For this review, take the finished solid that the model builds, in its own axes (mm). Face numbers are marked on the shaded views. A direction names the side the tool comes from. Round coordinates to 2 decimals unless told otherwise and drop trailing zeros. Order: outer loops, then holes, each group sorted by start corner. A loop starts at its lowest first (then second) coordinate and runs counter-clockwise, first axis right, second up. Notation, with made-up numbers: (54.25, 26.5) - (100.25, 26.5) arc R17 ccw to (100.25, 58.5) - close; hole circle Ø8 at (12, 7). An arc over 180 degrees is marked (long way). Write each question's results on one line, items separated by ' | '. Start each with the question number.
(1) Take a section at D-D, the plane y = -18. Give the boundary of the cut face in (x, z).
(2) Insertion check: pin 1 Ø1 at (y, z) = (2.5, 9) entering from +X; pin 2 Ø1 at (x, z) = (-17.5, 9) entering from -Y; pin 3 Ø1.5 at (x, y) = (5, -10) entering from -Z; pin 4 Ø3 at (x, z) = (-1.5, 5) entering from +Y. Each pin has a flat end and moves straight along its axis. Give the tip position at first contact, or say it passes through.
(3) Take a section at A-A, the plane x = 0. Give the boundary of the cut face in (y, z), plus the area to 3 significant figures.
(4) Take a section at C-C, the plane z = 10.75. Give the boundary of the cut face in (x, y), plus the area to 3 significant figures.
(5) For the marked faces 1, 2 and 3, list the 3-axis set-ups (+Z, -Z, +X, -X, +Y, -Y) from which the entire face can be reached by the end or side of a thin tool; tool diameter is ignored.
(6) Draft analysis for pull direction X (two halves, no side actions). For the marked faces 4, 5 and 6, state which applies: pulls with the +X half, pulls with the -X half, needs draft (parallel to the pull), parting line crosses it, or undercut.
(7) Take a section at B-B, the plane z = 1.25. Give the boundary of the cut face in (x, y), plus the area to 3 significant figures.
(8) For L1, parallel to Y at x = 0, z = 7; L2, parallel to Y at x = -0.5, z = 5; L3, parallel to Y at x = -8.5, z = 7.5, list the stretches that pass through material, from the lowest coordinate up. Write a range as from..to.
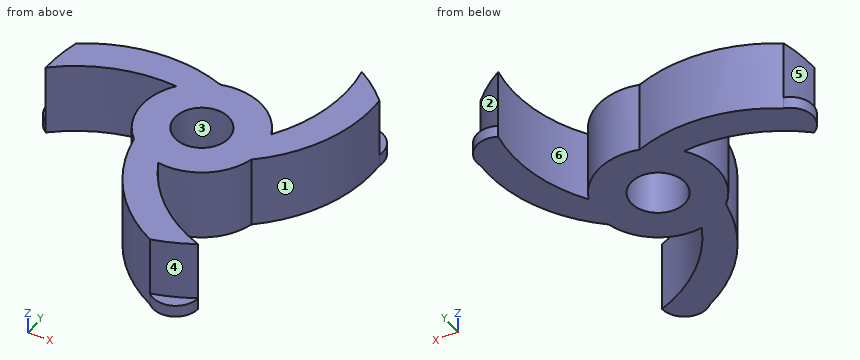
```python
from build123d import *

# Parameters (mm, degrees)
F0_R     = 4.5
F1_DEPTH = 12
F2_DEPTH = 2


with BuildPart() as f1:
    # F0 (on Top) → F1 (new body)
    with BuildSketch(Plane.XY):
        with BuildLine():
            ThreePointArc((-7.85878, 6.183815), (-5.508567, 8.345998), (-2.59656, 9.657012))
            ThreePointArc((-2.59656, 9.657012), (-14.056504, 11.131503), (-24.955515, 7.29536))
            ThreePointArc((-24.955515, 7.29536), (-25.706653, 3.894607), (-25.996543, 0.423975))
            ThreePointArc((-25.996543, 0.423975), (-17.497151, 5.097221), (-7.85878, 6.183815))
        make_face()
        with BuildLine():
            ThreePointArc((9.284731, 3.713996), (9.819555, 1.891122), (10, 0))
            ThreePointArc((10, 0), (9.915013, -1.300966), (9.661498, -2.579819))
            ThreePointArc((9.661498, -2.579819), (16.668417, 6.607538), (18.795724, 17.96443))
            ThreePointArc((18.795724, 17.96443), (16.226156, 20.315311), (13.365445, 22.301679))
            ThreePointArc((13.365445, 22.301679), (13.162898, 12.604367), (9.284731, 3.713996))
        make_face()
        with BuildLine():
            ThreePointArc((9.661498, -2.579819), (9.915013, -1.300966), (10, 0))
            ThreePointArc((10, 0), (9.819555, 1.891122), (9.284731, 3.713996))
            ThreePointArc((9.284731, 3.713996), (4.473563, 8.943558), (-2.59656, 9.657012))
            ThreePointArc((-2.59656, 9.657012), (-5.508567, 8.345998), (-7.85878, 6.183815))
            ThreePointArc((-7.85878, 6.183815), (-9.98213, -0.59756), (-7.064937, -7.077193))
            ThreePointArc((-7.064937, -7.077193), (-4.473563, -8.943558), (-1.425951, -9.897811))
            ThreePointArc((-1.425951, -9.897811), (5.508567, -8.345998), (9.661498, -2.579819))
        make_face()
        Circle(F0_R, mode=Mode.SUBTRACT)
        with BuildLine():
            ThreePointArc((12.631098, -22.725654), (4.334253, -17.701588), (-1.425951, -9.897811))
            ThreePointArc((-1.425951, -9.897811), (-4.473563, -8.943558), (-7.064937, -7.077193))
            ThreePointArc((-7.064937, -7.077193), (-2.611913, -17.739041), (6.159791, -25.25979))
            ThreePointArc((6.159791, -25.25979), (9.480498, -24.209919), (12.631098, -22.725654))
        make_face()
    extrude(amount=F1_DEPTH)

    # F0 (on Top) → F2 (join)
    with BuildSketch(Plane.XY):
        with BuildLine():
            ThreePointArc((-25.996543, 0.423975), (-25.706653, 3.894607), (-24.955515, 7.29536))
            ThreePointArc((-24.955515, 7.29536), (-27.674447, 4.192732), (-25.996543, 0.423975))
        make_face()
        with BuildLine():
            ThreePointArc((6.159791, -25.25979), (10.206211, -26.06314), (12.631098, -22.725654))
            ThreePointArc((12.631098, -22.725654), (9.480498, -24.209919), (6.159791, -25.25979))
        make_face()
        with BuildLine():
            ThreePointArc((18.795724, 17.96443), (17.468236, 21.870408), (13.365445, 22.301679))
            ThreePointArc((13.365445, 22.301679), (16.226156, 20.315311), (18.795724, 17.96443))
        make_face()
    extrude(amount=F2_DEPTH)


solid = f1.part
```
Results below:
1) outline: (-2.42, 0) - (4.67, 0) - (4.67, 12) - (-2.42, 12) - close
2) pin 1: stops at x = 14.69 | pin 2: stops at y = 4.93 | pin 3: passes through | pin 4: stops at y = 10
3) outline: (-20.78, 0) - (-12.51, 0) - (-12.51, 12) - (-20.78, 12) - close; (-10, 0) - (-4.5, 0) - (-4.5, 12) - (-10, 12) - close; (4.5, 0) - (10, 0) - (10, 12) - (4.5, 12) - close | area: 231 mm^2
4) outline: (-26, 0.42) arc R25 cw to (-7.86, 6.18) arc R10 ccw to (-7.06, -7.08) arc R25 ccw to (6.16, -25.26) arc R26 ccw to (12.63, -22.73) arc R25 cw to (-1.43, -9.9) arc R10 ccw to (9.66, -2.58) arc R25 ccw to (18.8, 17.96) arc R26 ccw to (13.37, 22.3) arc R25 cw to (9.28, 3.71) arc R10 ccw to (-2.6, 9.66) arc R25 ccw to (-24.96, 7.3) arc R26 ccw to start; hole circle Ø9 at (0, 0) | area: 572 mm^2
5) face 1: +Z, -Z, +X | face 2: +Z, +X, +Y | face 3: +Z, -Z
6) face 4: pulls with the +X half | face 5: pulls with the -X half | face 6: undercut
7) outline: (-26, 0.42) arc R25 cw to (-7.86, 6.18) arc R10 ccw to (-7.06, -7.08) arc R25 ccw to (6.16, -25.26) arc R3.83 ccw to (12.63, -22.73) arc R25 cw to (-1.43, -9.9) arc R10 ccw to (9.66, -2.58) arc R25 ccw to (18.8, 17.96) arc R3.83 ccw to (13.37, 22.3) arc R25 cw to (9.28, 3.71) arc R10 ccw to (-2.6, 9.66) arc R25 ccw to (-24.96, 7.3) arc R3.83 ccw to start; hole circle Ø9 at (0, 0) | area: 602 mm^2
8) L1: y = -20.78..-12.51, -10..-4.5, 4.5..10 | L2: y = -20.27..-11.67, -9.99..-4.47, 4.47..9.99 | L3: y = -5.27..5.27, 6.23..11.1
